Could you check a few things on this model? Use its own coordinates, in mm. Face numbers are marked on the shaded views. A direction names the side the tool comes from. Round coordinates to 2 decimals unless told otherwise and drop trailing zeros. Loops run counter-clockwise (first coordinate to the right, second up) from the corner with the lowest first, then second, coordinate; pieces in that order, holes last. Notation, with made-up numbers: M -14,69 L 10,69 A10 ccw 10,77 Z; hole C 19.25,83.25 d6. An arc over 180 degrees is marked long. Return JSON: item names as keys, results as strings. Group by question number.
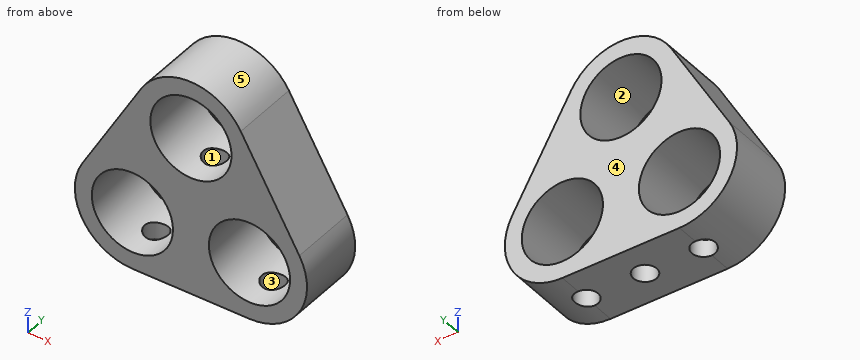
```python
from build123d import *

# Parameters (mm, degrees)
SKETCH1_W                       = 63.925633075
SKETCH1_H                       = 55.87744186
EXTRUDE1_DEPTH                  = 6.35
SKETCH2_OUTSIDE_W               = 82.953
SKETCH2_OUTSIDE_H               = 74.905
SKETCH2_OUTSIDE_R               = 3.8
CUT_EXTRUDE1_DEPTH              = 6.35
F_2_56_TAPPED_HOLE1_D           = 1.778
F_2_56_TAPPED_HOLE1_DEPTH       = 5.588
F_2_56_TAPPED_HOLE1_CBORE_D     = 2.1844
F_2_56_TAPPED_HOLE1_CBORE_DEPTH = 4.318
F_2_56_TAPPED_HOLE1_TIP         = 0.53416509
F_2_56_TAPPED_HOLE2_D           = 1.778
F_2_56_TAPPED_HOLE2_DEPTH       = 13.208
F_2_56_TAPPED_HOLE2_CBORE_D     = 2.1844
F_2_56_TAPPED_HOLE2_CBORE_DEPTH = 11.938
F_2_56_TAPPED_HOLE2_TIP         = 0.53416509


with BuildPart() as part:
    # Sketch1 → Extrude1 (new body)
    with BuildSketch(Plane(origin=(0, 0, 0), x_dir=(1, 0, 0), z_dir=(0, 1, 0))):
        with Locations((1.954560723, 3.334250646)):
            Rectangle(SKETCH1_W, SKETCH1_H)
    extrude(amount=EXTRUDE1_DEPTH)

    # Sketch2 outside → Cut-Extrude1 (cut)
    with BuildSketch(Plane.XZ):
        with Locations((1.9545, -3.3345)):
            Rectangle(SKETCH2_OUTSIDE_W, SKETCH2_OUTSIDE_H)
        with BuildLine():
            Line((-10.146711863, -0.470706825), (-4.665711863, 9.022663651))
            ThreePointArc((-4.665711863, 9.022663651), (0, 11.716413651), (4.665711863, 9.022663651))
            Line((4.665711863, 9.022663651), (10.146711863, -0.470706825))
            ThreePointArc((10.146711863, -0.470706825), (10.146711863, -5.858206825), (5.481, -8.551956825))
            Line((5.481, -8.551956825), (-5.481, -8.551956825))
            ThreePointArc((-5.481, -8.551956825), (-10.146711863, -5.858206825), (-10.146711863, -0.470706825))
        make_face(mode=Mode.SUBTRACT)
        with Locations((0, 6.328913651)):
            Circle(SKETCH2_OUTSIDE_R)
        with Locations((5.481, -3.164456825)):
            Circle(SKETCH2_OUTSIDE_R)
        with Locations((-5.481, -3.164456825)):
            Circle(SKETCH2_OUTSIDE_R)
    extrude(amount=-CUT_EXTRUDE1_DEPTH, mode=Mode.SUBTRACT)

    # #2-56 Tapped Hole1
    with Locations(Plane(origin=(5.481, 3.175, -8.551956825), x_dir=(-1, 0, 0), z_dir=(0, 0, -1))):
        with Locations((0, 0), (10.962, 0)):
            CounterBoreHole(F_2_56_TAPPED_HOLE1_D / 2, F_2_56_TAPPED_HOLE1_CBORE_D / 2, F_2_56_TAPPED_HOLE1_CBORE_DEPTH, depth=F_2_56_TAPPED_HOLE1_DEPTH)
            with Locations((0, 0, -(F_2_56_TAPPED_HOLE1_DEPTH + F_2_56_TAPPED_HOLE1_TIP / 2))):  # 118° drill point
                Cone(0, F_2_56_TAPPED_HOLE1_D / 2, F_2_56_TAPPED_HOLE1_TIP, mode=Mode.SUBTRACT)

    # #2-56 Tapped Hole2
    with Locations(Plane(origin=(0, 3.175, -8.551956825), x_dir=(-1, 0, 0), z_dir=(0, 0, -1))):
        with Locations((0, 0)):
            CounterBoreHole(F_2_56_TAPPED_HOLE2_D / 2, F_2_56_TAPPED_HOLE2_CBORE_D / 2, F_2_56_TAPPED_HOLE2_CBORE_DEPTH, depth=F_2_56_TAPPED_HOLE2_DEPTH)
            with Locations((0, 0, -(F_2_56_TAPPED_HOLE2_DEPTH + F_2_56_TAPPED_HOLE2_TIP / 2))):  # 118° drill point
                Cone(0, F_2_56_TAPPED_HOLE2_D / 2, F_2_56_TAPPED_HOLE2_TIP, mode=Mode.SUBTRACT)


solid = part.part
```
1. I'm going to push flat-ended pins straight in: pin 1 Ø7 at (x, z) = (-5.48, -3.16) entering from +Y; pin 2 Ø3 at (y, z) = (1.5, 0) entering from +X; pin 3 Ø1.5 at (y, z) = (4, -5) entering from +X; pin 4 Ø1.3 at (x, y) = (5.481, 3.175) entering from +Z. Where does each tip first touch, or does it pass through?
2. On a 3-axis mill with a long thin cutter (end or side, diameter ignored), from which of +Z, -Z, +X, -X, +Y, -Y can I reach the whole of each face in a straight line? I mean the marked faces 1 and 2. Say none if no direction works.
3. If we section it at A-A, the plane x = 0: Please give me the cut outline in (y, z).
4. I need wall thicknesses on probe 1 along Z at (x, y) = (0, 4.5); probe 2 along X at (y, z) = (3, -0.25); probe 3 along Y at (x, z) = (0, -4.5). Which ranges of each line are inside material? Lowest first, please.
5. If we section it at C-C, the plane y = 1.25: Please give me the cut outline in (x, z) (1 decimal), then the cut area to 3 significant figures.
6. We'd pull the mould along Y, two halves only. Please class the marked faces 3, 4 and 5: +Y half, -Y half, draft (parallel to the pull), parting line (faces both ways), or undercut.
7. If we section it at D-D, the plane z = 1.5: Please give me the cut outline in (x, y) (3 decimals).
8. If we section it at B-B, the plane z = 7.5: Please give me the cut outline in (x, y).
Geometry results:
{
 "1": {"pin 1": "through", "pin 2": "x = 10.6", "pin 3": "x = 10.76", "pin 4": "z = 8.74"},
 "2": {"face 1": "-Z", "face 2": "+Y, -Y"},
 "3": {"outline": "M 0,-8.55 L 2.08,-8.55 L 2.08,2.53 L 0,2.53 Z; M 0,10.13 L 6.35,10.13 L 6.35,11.72 L 0,11.72 Z; M 4.27,-8.55 L 6.35,-8.55 L 6.35,2.53 L 4.27,2.53 Z"},
 "4": {"probe 1": "-8.55 to 2.53, 10.13 to 11.72", "probe 2": "-10.02 to -7.92, -3.04 to -1.08, 1.08 to 3.04, 7.92 to 10.02", "probe 3": "0 to 2.08, 4.27 to 6.35"},
 "5": {"outline": "M -10.1,-0.5 A5.4 ccw -5.5,-8.6 L 5.5,-8.6 A5.4 ccw 10.1,-0.5 L 4.7,9 A5.4 ccw -4.7,9 Z; hole C -5.5,-3.2 d7.6; hole C 0,6.3 d7.6; hole C 5.5,-3.2 d7.6", "area": "184 mm^2"},
 "6": {"face 3": "undercut", "face 4": "+Y half", "face 5": "draft"},
 "7": {"outline": "M -9.009,0 L 9.009,0 L 9.009,6.35 L -9.009,6.35 Z; hole C 0,3.175 d2.184"},
 "8": {"outline": "M -5.54,0 L -3.62,0 L -3.62,6.35 L -5.54,6.35 Z; M 3.62,0 L 5.54,0 L 5.54,6.35 L 3.62,6.35 Z"}
}
